Read the model definition and answer for the solid it produces. Units are mm, in the model's axes. A direction names the side the tool comes from. Coordinates: 2 decimals unless noted, no trailing zeros. Order: outer loops, then holes, each group sorted by start corner. A loop starts at its lowest first (then second) coordinate and runs counter-clockwise, first axis right, second up. Notation, with made-up numbers: (-40, 56) -> (-21, 56) arc R30 cw to (-21, 82) -> close; hole circle Ø3 at (28.5, 6). An arc over 180 degrees is marked (long way). Answer as a JSON object with one key per item and string values. Group by question number.
1) A tool of negligible diameter and unlimited length cuts with its end or side. For faces 4 (the conical face through (0.84, -1.49, -0.12)), 5 (the flat face through (0, 0, -12.09)), 6 (the cylindrical face through (1.468, -1.915, -7.093)), from which of +Z, -Z, +X, -X, +Y, -Y can it reach the whole face along a straight path? Write none if from no direction.
2) Consider L1, parallel to Y at x = 0, z = -7.5; L2, parallel to Z at x = -3.75, y = -2.25; L3, parallel to X at y = 1, z = -0.25. Determine where each line is inside the solid, lowest interval first.
3) Given pin 1 (2.5 mm diameter, centred on x = -0.5, y = 0, fed in from +Z); pin 2 (2 mm diameter, centred on y = 2, z = -3, fed in from +X); pin 3 (1.5 mm diameter, centred on y = 2, z = -4.5, fed in from -X), each flat-ended and moving along its own axis, determine where each tip first touches the part or whether it passes through.
4) Determine the mould class of faces 1 (the cylindrical face through (4.476, 0.994, -2.376)), 2 (the conical face through (0.865, 1.473, -0.125)), 3 (the flat face through (-2, 0, 0)) for opening direction X: released by +X, released by -X, zero draft, split by the parting line, or undercut.
5) Section B-B on y = 3.5 is taken. Determine the outline of the cut face in (x, z).
6) Section A-A on z = -11 is taken. Determine the outline of the cut face in (x, y), and give its area (3 significant figures).
from build123d import *

# Parameters (mm, degrees)
SKETCH1_W          = 9.525
SKETCH1_H          = 2.413
CHAMFER1_SIZE      = 0.5953125
CUT_EXTRUDE2_DEPTH = 1.79578
SKETCH6_R          = 1.833087105
CUT_EXTRUDE3_DEPTH = 1.79578
CUT_EXTRUDE3_TAPER = 45


with BuildPart() as part:
    # Sketch1 → Revolve1 (revolve)
    with BuildSketch(Plane(origin=(0, 0, 0), x_dir=(0, 0, -1), z_dir=(1, 0, 0))):
        with Locations((7.3279, 1.2065)):
            Rectangle(SKETCH1_W, SKETCH1_H)
    revolve(axis=Axis((0, 0, -12.0904), (0, 0, 1)))

    # Chamfer1
    chamfer1_edges = [part.edges().sort_by_distance(p)[0] for p in [
        (0, -2.413, -12.0904),
    ]]
    chamfer(chamfer1_edges, length=CHAMFER1_SIZE)

    # Sketch7 → Revolve2 (revolve)
    with BuildSketch(Plane(origin=(0, 0, 0), x_dir=(0, 0, -1), z_dir=(1, 0, 0)), mode=Mode.PRIVATE) as revolve2_sk:
        with BuildLine():
            Line((2.18059, 4.5847), (2.5654, 4.5847))
            Line((2.5654, 4.5847), (2.5654, 0))
            Line((2.5654, 0), (0, 0))
            Line((0, 0), (0, 2.413))
            ThreePointArc((0, 2.413), (0.925030326, 3.664791196), (2.18059, 4.5847))
        make_face()
    revolve(revolve2_sk.sketch.rotate(Axis((0, 0, 0), (0, 0, -1)), 180), axis=Axis((0, 0, 0), (0, 0, -1)))

    # Sketch5 → Cut-Extrude2 (cut)
    with BuildSketch(Plane.XY):
        Polygon((1.5875, -0.916543552), (1.5875, 0.916543552), (0, 1.833087105), (-1.5875, 0.916543552), (-1.5875, -0.916543552), (0, -1.833087105), align=None)
    extrude(amount=-CUT_EXTRUDE2_DEPTH, mode=Mode.SUBTRACT)

    # Sketch6 → Cut-Extrude3 (cut)
    with BuildSketch(Plane.XY):
        Circle(SKETCH6_R)
    extrude(amount=-CUT_EXTRUDE3_DEPTH, taper=CUT_EXTRUDE3_TAPER, mode=Mode.SUBTRACT)


solid = part.part
Worked answers:
{
 "1": {"face 4": "+Z", "face 5": "-Z, +X, -X, +Y, -Y", "face 6": "-Z"},
 "2": {"L1": "y = -2.41 to 2.41", "L2": "z = -2.57 to -1.81", "L3": "x = -2.65 to -1.44, 1.44 to 2.65"},
 "3": {"pin 1": "stops at z = -0.08", "pin 2": "stops at x = 4.45", "pin 3": "stops at x = -2.06"},
 "4": {"face 1": "split by the parting line", "face 2": "undercut", "face 3": "zero draft"},
 "5": {"outline": "(-2.96, -2.57) -> (2.96, -2.57) -> (2.96, -2.18) arc R3.81 ccw to (-2.96, -2.18) -> close"},
 "6": {"outline": "circle Ø4.83 at (0, 0)", "area": "18.3 mm²"}
}
